from build123d import *

# Parameters (mm, degrees)
SKETCH1_W           = 129.7
SKETCH1_H           = 180
SKETCH1_R           = 2.5
SKETCH1_R_2         = 3.6
BOSS_EXTRUDE1_DEPTH = 5
FILLET1_R           = 3


with BuildPart() as part:
    # Sketch1 → Boss-Extrude1 (new body)
    with BuildSketch(Plane.XY):
        with Locations((64.85, 90)):
            Rectangle(SKETCH1_W, SKETCH1_H)
        with Locations((15, 15)):
            Circle(SKETCH1_R, mode=Mode.SUBTRACT)
        with Locations((15, 165)):
            Circle(SKETCH1_R, mode=Mode.SUBTRACT)
        with Locations((114.7, 165)):
            Circle(SKETCH1_R_2, mode=Mode.SUBTRACT)
        with Locations((114.7, 15)):
            Circle(SKETCH1_R_2, mode=Mode.SUBTRACT)
        with Locations((74.85, 90)):
            Circle(SKETCH1_R, mode=Mode.SUBTRACT)
        with Locations((54.85, 90)):
            Circle(SKETCH1_R, mode=Mode.SUBTRACT)
    extrude(amount=BOSS_EXTRUDE1_DEPTH)

    # Fillet1
    fillet1_edges = [part.edges().sort_by_distance(p)[0] for p in [
        (0, 180, 2.5),
        (129.7, 180, 2.5),
        (129.7, 0, 2.5),
        (0, 0, 2.5),
    ]]
    fillet(fillet1_edges, radius=FILLET1_R)


solid = part.part
Work out the finished part from the listing and answer in its coordinate system (mm). Round coordinates to 2 decimals unless told otherwise and drop trailing zeros. Order: outer loops, then holes, each group sorted by start corner. A loop starts at its lowest first (then second) coordinate and runs counter-clockwise, first axis right, second up. Notation, with made-up numbers: M 47.5,-26 L 54.5,-26 A27 ccw 54.5,8 Z; hole C -9.75,34.25 d8. An arc over 180 degrees is marked long. Put each result on its own line as item: value. Start each with the question number.
Q1. Section C-C, the plane x = 74.85 is taken. Write down the section's boundary in (y, z).
Q2. Straight lines are drawn through the part: L1, parallel to Y at x = 114.7, z = 1.6; L2, parallel to Y at x = 74.85, z = 2.65; L3, parallel to Y at x = 15, z = 1.7. For each, find the intervals that lie inside material, in ascending order. Write a range as [from, to].
Q3. Section B-B, the plane x = 114.7 is taken. Write down the section's boundary in (y, z), and give its area (3 significant figures).
Q4. A flat-ended cylindrical pin translates along its axis: pin 1 (6 mm diameter, centred on x = 24.5, y = 155, fed in from -Z). Find the tip coordinate at first contact, or state that the pin passes through.
Q5. For a pull along Y with two mould halves and no side action, classify faces 1 (the flat face through (64, 180, 2)), 2 (the cylindrical face through (77.235, 90.751, 2.465)), 3 (the flat face through (129.7, 89, 2)), 4 (the flat face through (64, 0, 2)) as pulls with the +Y half, pulls with the -Y half, needs draft (parallel to the pull), parting line crosses it, or undercut.
Q6. Section A-A, the plane y = 15 is taken. Write down the section's boundary in (x, z), and give its area (4 significant figures).
Findings below:
1. outline: M 0,0 L 87.5,0 L 87.5,5 L 0,5 Z; M 92.5,0 L 180,0 L 180,5 L 92.5,5 Z
2. L1: y = [0, 11.4], [18.6, 161.4], [168.6, 180]
2. L2: y = [0, 87.5], [92.5, 180]
2. L3: y = [0, 12.5], [17.5, 162.5], [167.5, 180]
3. outline: M 0,0 L 11.4,0 L 11.4,5 L 0,5 Z; M 18.6,0 L 161.4,0 L 161.4,5 L 18.6,5 Z; M 168.6,0 L 180,0 L 180,5 L 168.6,5 Z
3. area: 828 mm^2
4. pin 1: stops at z = 0
5. face 1: pulls with the +Y half
5. face 2: undercut
5. face 3: needs draft
5. face 4: pulls with the -Y half
6. outline: M 0,0 L 12.5,0 L 12.5,5 L 0,5 Z; M 17.5,0 L 111.1,0 L 111.1,5 L 17.5,5 Z; M 118.3,0 L 129.7,0 L 129.7,5 L 118.3,5 Z
6. area: 587.5 mm^2
